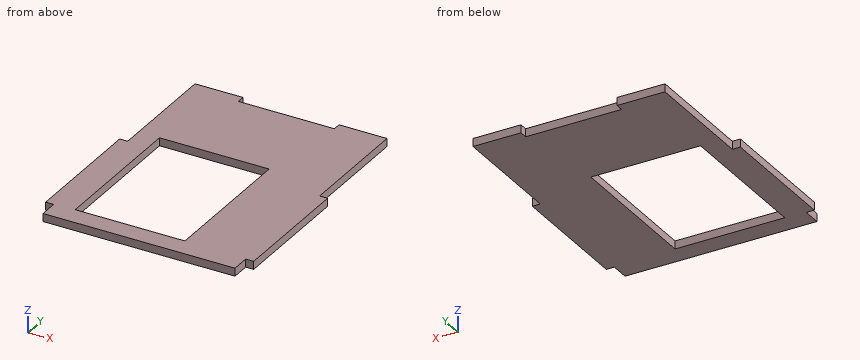
Autodesk Inventor part; units mm, degrees
ref_plane "YZ Plane" through (0, 0, 0) normal (1, 0, 0) x (0, 1, 0)
ref_plane "XZ Plane" through (0, 0, 0) normal (0, 1, 0) x (-1, 0, 0)
ref_plane "XY Plane" through (0, 0, 0) normal (0, 0, 1) x (1, 0, 0)
sketch "Sketch1" plane through (0, 0, 0) normal (0, 0, 1) x (1, 0, 0)
  line L0 (0, 0) -> (76.2, 0)
  line L1 (76.2, 0) -> (76.2, 79.0194)
  line L2 (76.2, 79.0194) -> (0, 79.0194)
  line L3 (0, 79.0194) -> (0, 0)
  line L4 (0, 7.3406) -> (-3.175, 7.3406)
  line L5 (-3.175, 7.3406) -> (-3.175, 58.1406)
  line L6 (-3.175, 58.1406) -> (0, 58.1406)
  line L7 (0, 58.1406) -> (0, 7.3406)
  line L8 (38.1, 79.0194) -> (38.1, 15.1376) construction
  line L9 (76.2, 0) -> (0, 0)
  line L10 (76.2, 79.0194) -> (76.2, 0)
  line L11 (76.2, 7.3406) -> (79.375, 7.3406)
  line L12 (79.375, 7.3406) -> (79.375, 58.1406)
  line L13 (79.375, 58.1406) -> (76.2, 58.1406)
  line L14 (76.2, 58.1406) -> (76.2, 7.3406)
  dimension "d0" = 76.2
  dimension "d1" = 79.0194
  dimension "d2" = 7.3406
  dimension "d3" = 50.8
  dimension "d6" = 3.175
extrude "Extrusion1" add sketch "Sketch1" along normal blind 3.175
sketch "Sketch2" plane through (0, 0, 3.175) normal (0, 0, 1) x (1, 0, 0)
  line L0 (76.2, 79.0194) -> (0, 79.0194)
  line L1 (0, 79.0194) -> (76.2, 79.0194)
  line L2 (76.2, 79.0194) -> (76.2, 104.4194)
  line L3 (76.2, 104.4194) -> (0, 104.4194)
  line L4 (0, 104.4194) -> (0, 79.0194)
  point P0 (0, 0)
  dimension "d7" = 25.4
extrude "Extrusion2" add sketch "Sketch2" against normal blind 3.175
sketch "Sketch3" plane through (0, 0, 3.175) normal (0, 0, 1) x (1, 0, 0)
  line L0 (76.2, 104.4194) -> (0, 104.4194)
  line L1 (19.05, 104.4194) -> (57.15, 104.4194)
  line L2 (57.15, 104.4194) -> (57.15, 101.2444)
  line L3 (57.15, 101.2444) -> (19.05, 101.2444)
  line L4 (19.05, 101.2444) -> (19.05, 104.4194)
  line L5 (0, 104.4194) -> (0, 58.1406)
  point P0 (0, 0)
  dimension "d10" = 3.175
  dimension "d11" = 38.1
  dimension "d12" = 19.05
extrude "Extrusion3" cut sketch "Sketch3" against normal blind 3.175
sketch "Sketch5" plane through (0, 0, 3.175) normal (0, 0, 1) x (1, 0, 0)
  line L0 (51.7909, 65.7282) -> (8.247, 65.7282)
  line L1 (8.247, 65.7282) -> (8.247, 7.8346)
  line L2 (8.247, 7.8346) -> (51.7909, 7.8346)
  line L3 (51.7909, 7.8346) -> (51.7909, 65.7282)
  point P0 (0, 0)
extrude "Extrusion4" cut sketch "Sketch5" against normal blind 25.4
properties part number "front"
The model under review builds one solid part; all positions refer to its coordinate system, in mm. Round coordinates to 2 decimals unless told otherwise and drop trailing zeros. Write each loop counter-clockwise with the first axis right and the second up, starting at its lowest first coordinate (ties: lowest second). Pieces come first, ordered by that corner, then holes. Notation, with made-up numbers: M 76.5,76.25 L 102.5,76.25 A16 ccw 102.5,85.25 Z; hole C 60,-33 d10. An arc over 180 degrees is marked long. Use CSV: the item, a comma, the result in double quotes. Start each with the question number.
(1) We need section D-D, the plane y = 97. State the section outline as (x, z) points (3 decimals).
(2) For line 1 along Y through (x, z) = (33, 2.95); line 2 along Y through (x, z) = (9, 2.35); line 3 along X through (y, z) = (47, 1.1) (3 decimals), list the stretches that pass through material, from the lowest coordinate up.
(3) We need section C-C, the plane z = 0.75. State the section outline as (x, y) points (3 decimals).
(4) We need section B-B, the plane y = 17.5. State the section outline as (x, z) points (3 decimals).
(5) Clearance check with flat-ended pins moving along their axes: P1, Ø1, axis at y = 5.5, z = 2, coming from the +X side; P2, Ø1.6, axis at x = -1.5, z = 2, coming from the -Y side; P3, Ø1, axis at y = 80.5, z = 1, coming from the -X side; P4, Ø12, axis at x = 6, y = 45.5, coming from the -Z side. State where each tip first meets the part, or that it passes through.
(6) We need section A-A, the plane x = 13. State the section outline as (y, z) points (3 decimals), then the cut area to 3 significant figures.
Findings:
1,outline,"M 0,0 L 76.2,0 L 76.2,3.175 L 0,3.175 Z"
2,line 1,"0 to 7.83, 65.73 to 101.24"
2,line 2,"0 to 7.83, 65.73 to 104.42"
2,line 3,"-3.175 to 8.247, 51.791 to 79.375"
3,outline,"M -3.175,7.341 L 0,7.341 L 0,0 L 76.2,0 L 76.2,7.341 L 79.375,7.341 L 79.375,58.141 L 76.2,58.141 L 76.2,104.419 L 57.15,104.419 L 57.15,101.244 L 19.05,101.244 L 19.05,104.419 L 0,104.419 L 0,58.141 L -3.175,58.141 Z; hole M 8.247,7.835 L 51.791,7.835 L 51.791,65.728 L 8.247,65.728 Z"
4,outline,"M -3.175,0 L 8.247,0 L 8.247,3.175 L -3.175,3.175 Z; M 51.791,0 L 79.375,0 L 79.375,3.175 L 51.791,3.175 Z"
5,P1,"x = 76.2"
5,P2,"y = 7.34"
5,P3,"x = 0"
5,P4,"z = 0"
6,outline,"M 0,0 L 7.835,0 L 7.835,3.175 L 0,3.175 Z; M 65.728,0 L 104.419,0 L 104.419,3.175 L 65.728,3.175 Z"
6,area,"148 mm^2"
